Build history of the part. All positions in model axes, mm. A direction names the side the tool comes from. Give positions to 0.01 mm unless a question says otherwise; leave off trailing zeros. Loops run counter-clockwise (first coordinate to the right, second up) from the corner with the lowest first, then second, coordinate; pieces in that order, holes last. Notation, with made-up numbers: (-25.75, 33.25) - (-15.75, 33.25) arc R11 ccw to (-15.75, 49.25) - close; hole circle Ø7 at (-25, 89.5). An arc over 180 degrees is marked (long way). Return JSON: item names as keys, results as strings. Group by question number.
1) 3-axis set-ups, long thin cutter, end or side, ignore diameter. For faces 4 (the face through (2, -2, 14)), 5 (the face through (4.006, 1.262, 10.451)): which of +Z, -Z, +X, -X, +Y, -Y reach the whole face in a straight line?
2) Slice it at A-A (x = 0). List the corners of the cut face in (y, z).
3) Mould opens along Y. For faces 1 (the face through (6, 0, 0)), 2 (the face through (-29.97, 1.32, 0.38)), 3 (the face through (10, 0, 2)) say: released by +Y, released by -Y, zero draft, split by the parting line, or undercut.
4) Drop flat-ended pins along their axis: pin 1 (1 mm diameter, centred on x = -1, y = -7, fed in from +Z); pin 2 (1.5 mm diameter, centred on x = 22, z = 11, fed in from -Y); pin 3 (6 mm diameter, centred on x = 6, y = -18, fed in from +Z). Give the stop position or say it passes through.
5) Drill centre lines: probe 1 along Y at (x, z) = (0, 7); probe 2 along Y at (x, z) = (0, 9.5); probe 3 along Z at (x, y) = (-11, 3.5). Where is each one in solid material? Low to high. Write a range as from..to.
6) Slice it at B-B (z = 12.5). List the corners of the cut face in (x, y).
```python
from build123d import *

# Parameters (mm, degrees)
F0_R     = 30
F0_R_2   = 2.2
F1_DEPTH = 14
F2_T     = -2
F3_SIZE  = 5
F4_R     = 3


with BuildPart() as f1:
    # F0 (on Top) → F1 (new body)
    with BuildSketch(Plane.XY):
        Circle(F0_R)
        Circle(F0_R_2, mode=Mode.SUBTRACT)
    extrude(amount=F1_DEPTH)

    # F2
    f2_openings = [f1.faces().sort_by_distance(p)[0] for p in [
        (-29.151472, 0, 14),
    ]]
    offset(amount=F2_T, openings=f2_openings)

    # F3
    f3_edges = [f1.edges().sort_by_distance(p)[0] for p in [
        (-28, 0, 2),
        (-4.2, 0, 2),
    ]]
    chamfer(f3_edges, length=F3_SIZE)

    # F5: sweep along a path in F5_path
    with BuildLine(Plane(origin=(30, 0, 14), x_dir=(0, -1, 0), z_dir=(0, 0, -1))) as f5_path:
        CenterArc((0, 30), 30, 0, 360)
    # F4 (on Front) → F5 (sweep, cut)
    with BuildSketch(Plane.XZ):
        with Locations((-32, 2.9998219346)):
            Circle(F4_R)
        with Locations((-31.9502516922, 11)):
            Circle(F4_R)
    sweep(path=f5_path.line, mode=Mode.SUBTRACT)


solid = f1.part
```
Results:
{
 "1": {"face 4": "+Z, +X, -X, +Y, -Y", "face 5": "+Z"},
 "2": {"outline": "(-30, 0) - (-2.2, 0) - (-2.2, 14) - (-4.2, 14) - (-4.2, 7) - (-9.2, 2) - (-23, 2) - (-28, 7) - (-28, 14) - (-30, 14) - (-30, 13.28) arc R3 cw to (-30, 8.72) - (-30, 5.24) arc R3 cw to (-30, 0.76) - close; (2.2, 0) - (30, 0) - (30, 0.76) arc R3 cw to (30, 5.24) - (30, 8.72) arc R3 cw to (30, 13.28) - (30, 14) - (28, 14) - (28, 7) - (23, 2) - (9.2, 2) - (4.2, 7) - (4.2, 14) - (2.2, 14) - close"},
 "3": {"face 1": "zero draft", "face 2": "split by the parting line", "face 3": "undercut"},
 "4": {"pin 1": "z = 4.63", "pin 2": "y = -19.66", "pin 3": "z = 2"},
 "5": {"probe 1": "-30..-28, -4.2..-2.2, 2.2..4.2, 28..30", "probe 2": "-29.35..-28, -4.2..-2.2, 2.2..4.2, 28..29.35", "probe 3": "0..2"},
 "6": {"outline": "circle Ø58.7 at (0, 0); circle Ø8.4 at (0, 0); hole circle Ø56 at (0, 0); hole circle Ø4.4 at (0, 0)"}
}
